Geometry check sheet. Reference: drawing and pictorial views, mm from the part's lowest x, y, z. A direction names the side the tool comes from. Give positions to 0.01 mm unless a question says otherwise; leave off trailing zeros. Write each loop counter-clockwise with the first axis right and the second up, starting at its lowest first coordinate (ties: lowest second). Pieces come first, ordered by that corner, then holes. Notation, with made-up numbers: (-22, -10.75) -> (14, -10.75) arc R28 cw to (14, 14.25) -> close; hole circle Ø9 at (56.25, 84.5). An arc over 180 degrees is marked (long way). Return JSON: item names as keys, results as strings.
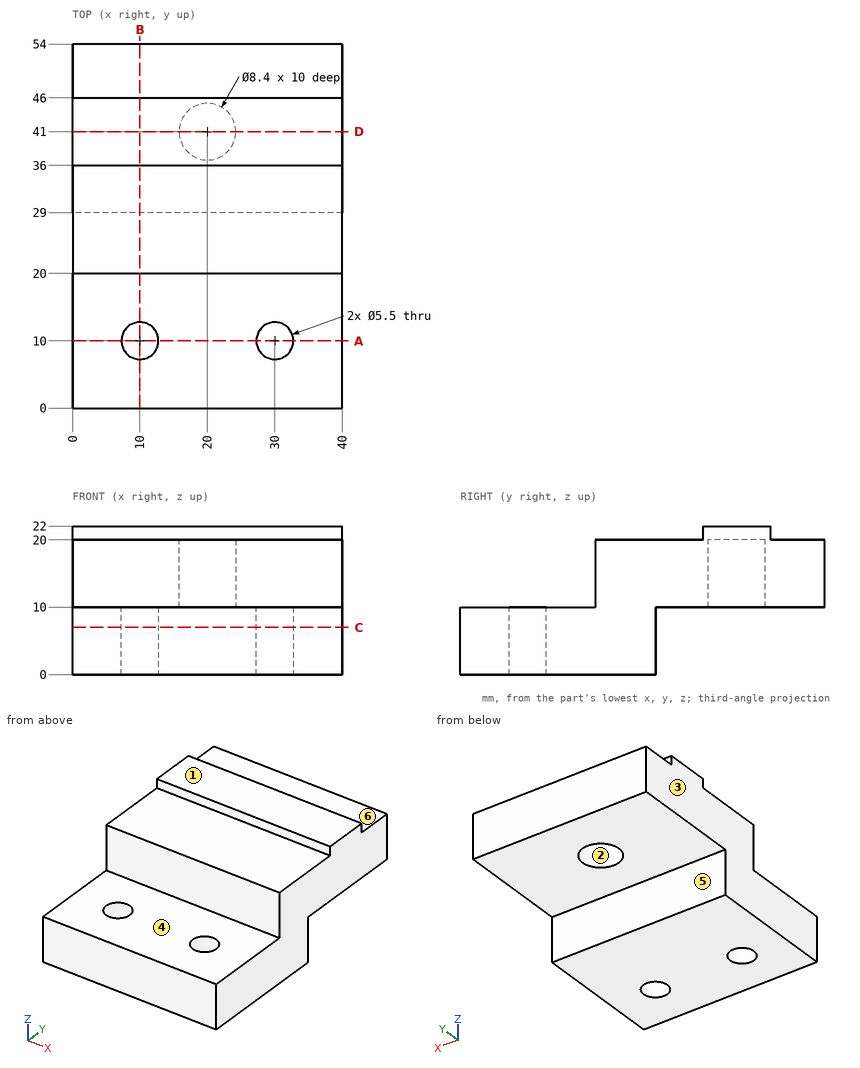
(1) Set-up check for the marked faces 4, 5 and 6: record each of +Z, -Z, +X, -X, +Y, -Y from which the full face is reachable in a straight line by a thin tool's end or side.
Reply:
{"face 4": "+Z, +X, -X, -Y", "face 5": "-Z, +X, -X, +Y", "face 6": "+Z, +X, -X, +Y"}
(2) Cross-section at C-C on z = 7. Enter the section's corners in (x, y), then the cut area to 3 significant figures.
Reply:
{"outline": "(0, 0) -> (40, 0) -> (40, 29) -> (0, 29) -> close; hole circle Ø5.5 at (10, 10); hole circle Ø5.5 at (30, 10)", "area": "1,110 mm^2"}
(3) Thickness scan on L1, parallel to Y at x = 30, z = 2.5; L2, parallel to Y at x = 20, z = 16; L3, parallel to Z at x = 36.5, y = 34. Record the ranges inside material, lowest first.
Reply:
{"L1": "0 to 7.25, 12.75 to 29", "L2": "20 to 36.8, 45.2 to 54", "L3": "10 to 20"}
(4) Release check for a two-part mould opening along X. For the marked faces 1, 2 and 3 record: pulls with the +X half, pulls with the -X half, needs draft (parallel to the pull), parting line crosses it, or undercut.
Reply:
{"face 1": "needs draft", "face 2": "undercut", "face 3": "pulls with the -X half"}
(5) Cross-section at A-A on y = 10. Enter the section's corners in (x, z).
Reply:
{"outline": "(0, 0) -> (7.25, 0) -> (7.25, 10) -> (0, 10) -> close; (12.75, 0) -> (27.25, 0) -> (27.25, 10) -> (12.75, 10) -> close; (32.75, 0) -> (40, 0) -> (40, 10) -> (32.75, 10) -> close"}
(6) Cross-section at B-B on x = 10. Enter the section's corners in (y, z).
Reply:
{"outline": "(0, 0) -> (7.25, 0) -> (7.25, 10) -> (0, 10) -> close; (12.75, 0) -> (29, 0) -> (29, 10) -> (54, 10) -> (54, 20) -> (46, 20) -> (46, 22) -> (36, 22) -> (36, 20) -> (20, 20) -> (20, 10) -> (12.75, 10) -> close"}
(7) Depth check by flat-ended pin: pin 1 Ø6 at (x, y) = (13, 7) entering from +Z; pin 2 Ø5 at (x, y) = (10, 10) entering from +Z; pin 3 Ø8 at (x, z) = (21, 3) entering from +Y; pin 4 Ø8 at (x, z) = (26.5, 16) entering from -Y. Enter the tip coordinate at first touch or a pass-through.
Reply:
{"pin 1": "z = 10", "pin 2": "through", "pin 3": "y = 29", "pin 4": "y = 20"}
(8) Cross-section at D-D on y = 41. Enter the section's corners in (x, z).
Reply:
{"outline": "(0, 10) -> (15.8, 10) -> (15.8, 20) -> (24.2, 20) -> (24.2, 10) -> (40, 10) -> (40, 22) -> (0, 22) -> close"}
